The model under review builds one solid part; all positions refer to its coordinate system, in mm. A direction names the side the tool comes from. Coordinates: 2 decimals unless noted, no trailing zeros. Loops run counter-clockwise (first coordinate to the right, second up) from the corner with the lowest first, then second, coordinate; pieces in that order, holes last. Notation, with made-up numbers: M 82,12.5 L 137,12.5 A20 ccw 137,46.5 Z; hole C -23.5,79 d10. An arc over 180 degrees is marked long. Return JSON: item names as keys, results as strings.
```python
from build123d import *

# Parameters (mm, degrees)
SKETCH1_W           = 19.8
SKETCH1_H           = 4.9
BOSS_EXTRUDE1_DEPTH = 30
SKETCH2_W           = 9.9
SKETCH2_H           = 4.9
BOSS_EXTRUDE2_DEPTH = 10


with BuildPart() as part:
    # Sketch1 → Boss-Extrude1 (new, symmetric)
    with BuildSketch(Plane(origin=(0, 0, 0), x_dir=(0, 0, -1), z_dir=(1, 0, 0))):
        Rectangle(SKETCH1_W, SKETCH1_H)
    extrude(amount=BOSS_EXTRUDE1_DEPTH, both=True)

    # Sketch2 → Boss-Extrude2 (add)
    with BuildSketch(Plane(origin=(30, 0, 0), x_dir=(0, 0, -1), z_dir=(1, 0, 0))):
        Rectangle(SKETCH2_W, SKETCH2_H)
    boss_extrude2 = extrude(amount=BOSS_EXTRUDE2_DEPTH)

    # Mirror1: Boss-Extrude2 across plane
    add(boss_extrude2.mirror(Plane(origin=(0, 0, 0), x_dir=(0, 0, 1), z_dir=(1, 0, 0))))


solid = part.part
```
1. Insertion check: pin 1 Ø2 at (y, z) = (1.5, 8) entering from -X; pin 2 Ø2.5 at (y, z) = (-1, -7.5) entering from +X; pin 3 Ø2.5 at (x, y) = (-34, -0.5) entering from -Z. Each pin has a flat end and moves straight along its axis. Give the tip position at first contact, or say it passes through.
Check values:
{"pin 1": "x = -30", "pin 2": "x = 30", "pin 3": "z = -4.95"}
2. Add section B-B on z = 8.75. Give the boundary of the cut face in (x, y), plus the area to 3 significant figures.
Check values:
{"outline": "M -30,-2.45 L 30,-2.45 L 30,2.45 L -30,2.45 Z", "area": "294 mm²"}
3. Add section A-A on y = -1.25. Give the boundary of the cut face in (x, z), plus the area to 3 significant figures.
Check values:
{"outline": "M -40,-4.95 L -30,-4.95 L -30,-9.9 L 30,-9.9 L 30,-4.95 L 40,-4.95 L 40,4.95 L 30,4.95 L 30,9.9 L -30,9.9 L -30,4.95 L -40,4.95 Z", "area": "1,390 mm²"}
4. To check wall thickness, follow line 1 (X direction, y = -2.1, z = -8); line 2 (Z direction, x = 37.5, y = -0.45). State the ranges of each line that lie inside material, in increasing order.
Check values:
{"line 1": "-30 to 30", "line 2": "-4.95 to 4.95"}
5. Add section C-C on x = 33. Give the boundary of the cut face in (y, z), plus the area to 3 significant figures.
Check values:
{"outline": "M -2.45,-4.95 L 2.45,-4.95 L 2.45,4.95 L -2.45,4.95 Z", "area": "48.5 mm²"}
6. Machinability: for faces 1 (the face through (35, 0, -4.95)), 2 (the face through (-30, 0, -7)), 3 (the face through (-30, 0, 7)), 4 (the face through (30, 0, 7)), which of the approach directions +Z, -Z, +X, -X, +Y, -Y give a long, thin tool a straight path to every point of the face, cutting with its end or side? Answer none if there is none.
Check values:
{"face 1": "-Z, +X, +Y, -Y", "face 2": "-Z, -X, +Y, -Y", "face 3": "+Z, -X, +Y, -Y", "face 4": "+Z, +X, +Y, -Y"}
